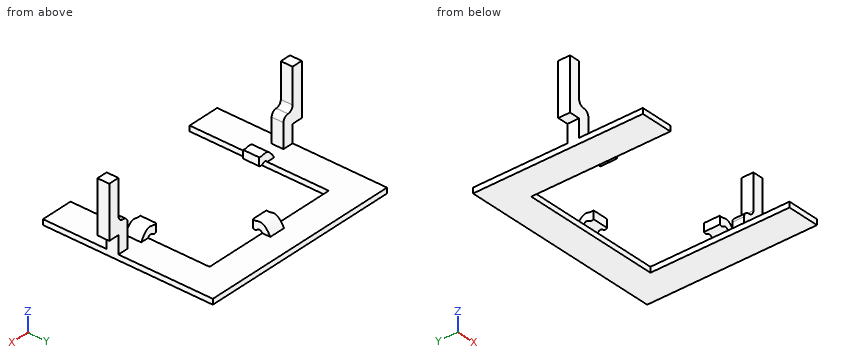
from build123d import *

# Parameters (mm, degrees)
BOSS_EXTRUDE1_DEPTH      = 1
BOSS_EXTRUDE2_START      = -1.5
BOSS_EXTRUDE2_DEPTH      = 3
CIRPATTERN1_COUNT        = 3
CIRPATTERN1_ANGLE        = 180
SKETCH4_W                = 2
SKETCH4_H                = 2.2
BOSS_EXTRUDE3_DEPTH      = 5.5
BOSS_EXTRUDE4_DEPTH      = 7.5
BOSS_EXTRUDE4_DEPTH_BACK = 2.2
SKETCH5_W                = 2
SKETCH5_H                = 2.2
FILLET1_START            = -30
FILLET1_DEPTH            = 4
FILLET1_START_2          = -29.415
FILLET1_2_DEPTH          = 2.2


with BuildPart() as part:
    # Sketch1 → Boss-Extrude1 (new body)
    with BuildSketch(Plane.XY):
        Polygon((13, -9.565), (-13, -9.565), (-19, -9.565), (-19, -41.315), (-13, -41.315), (-13, -15.315), (13, -15.315), (13, -41.315), (19, -41.315), (19, -9.565), align=None)
    extrude(amount=BOSS_EXTRUDE1_DEPTH)

    # Boss-Extrude2: read off the stored shape, not the designer's step
    # Boss-Extrude2 outline → Boss-Extrude2 (add)
    with BuildSketch(Plane(origin=(0, -28.315, 0), x_dir=(-1, 0, 0), z_dir=(0, -1, 0)).offset(BOSS_EXTRUDE2_START)):
        with BuildLine():
            Line((-11.23522271, -2.644286359), (-11.23522271, -1.144286359))
            add(Edge.make_bspline(
                [(-11.23522271, -1.144286359), (-11.740174878, -0.757764956), (-12.028679887, -1.161534837), (-12.227869222, -1.503002268), (-12.747184273, -1.488774458), (-13, -1)],
                knots=[0, 0, 0, 0, 0, 0, 1, 1, 1, 1, 1, 1], degree=5))
            Line((-13, -1), (-14.5, -1))
            add(Edge.make_bspline(
                [(-14.5, -1), (-13.760887065, -2.414906572), (-12.67824158, -3.40768712), (-12.345095428, -2.525951835), (-11.7215069, -2.450856602), (-11.23522271, -2.644286359)],
                knots=[0, 0, 0, 0, 0, 0, 1, 1, 1, 1, 1, 1], degree=5))
        make_face()
    boss_extrude2 = extrude(amount=BOSS_EXTRUDE2_DEPTH)

    # CirPattern1: Boss-Extrude2 ×3 about axis
    cirpattern1_axis = Axis((0, -28.315, 1.05), (0, 0, 1))
    for i in range(1, CIRPATTERN1_COUNT):
        add(boss_extrude2.rotate(cirpattern1_axis, i * CIRPATTERN1_ANGLE / (CIRPATTERN1_COUNT - 1)))

    # Sketch4 → Boss-Extrude3 (add)
    with BuildSketch(Plane.XY.offset(1)):
        with Locations((-18, -28.315)):
            Rectangle(SKETCH4_W, SKETCH4_H)
        with Locations((18, -28.315)):
            Rectangle(SKETCH4_W, SKETCH4_H)
    extrude(amount=BOSS_EXTRUDE3_DEPTH)

    # Sketch5 → Boss-Extrude4 (add, two sides: drawn at the far end of the back side and taken through both)
    with BuildSketch(Plane.XY.offset(6.5).offset(-BOSS_EXTRUDE4_DEPTH_BACK)):
        with Locations((-20, -28.315)):
            Rectangle(SKETCH5_W, SKETCH5_H)
        with Locations((20, -28.315)):
            Rectangle(SKETCH5_W, SKETCH5_H)
    extrude(amount=BOSS_EXTRUDE4_DEPTH + BOSS_EXTRUDE4_DEPTH_BACK)

    # Fillet1: read off the stored shape, not the designer's step
    # Fillet1 outline → Fillet1 (cut)
    with BuildSketch(Plane(origin=(0, 0, 0), x_dir=(1, 0, 0), z_dir=(0, 1, 0)).offset(FILLET1_START)):
        with BuildLine():
            Line((17, -6.5), (18, -6.5))
            ThreePointArc((18, -6.5), (17.292893219, -6.207106781), (17, -5.5))
            Line((17, -5.5), (17, -6.5))
        make_face()
        with BuildLine():
            ThreePointArc((-17, -5.5), (-17.292893219, -6.207106781), (-18, -6.5))
            Line((-18, -6.5), (-17, -6.5))
            Line((-17, -6.5), (-17, -5.5))
        make_face()
    extrude(amount=FILLET1_DEPTH, mode=Mode.SUBTRACT)

    # Fillet1 2 outline → Fillet1 2 (add)
    with BuildSketch(Plane(origin=(0, 0, 0), x_dir=(1, 0, 0), z_dir=(0, 1, 0)).offset(FILLET1_START_2)):
        with BuildLine():
            Line((19, -6.5), (18, -6.5))
            ThreePointArc((18, -6.5), (18.707106781, -6.792893219), (19, -7.5))
            Line((19, -7.5), (19, -6.5))
        make_face()
        with BuildLine():
            ThreePointArc((-19, -7.5), (-18.707106781, -6.792893219), (-18, -6.5))
            Line((-18, -6.5), (-19, -6.5))
            Line((-19, -6.5), (-19, -7.5))
        make_face()
    extrude(amount=FILLET1_2_DEPTH)


solid = part.part
Geometry: final body of the model. Coordinates: model frame, mm. Give positions to 0.01 mm unless a question says otherwise; leave off trailing zeros. Loops run counter-clockwise (first coordinate to the right, second up) from the corner with the lowest first, then second, coordinate; pieces in that order, holes last. Notation, with made-up numbers: M 77,79.25 L 101,79.25 A30 ccw 101,107.25 Z; hole C 47.5,-14 d2. An arc over 180 degrees is marked long. Put each result on its own line as item: value.
1) Material intervals for L1, parallel to X at y = -28.5, z = 5.5; L2, parallel to Z at x = 15, y = -18, sorted ascending. Write a range as from..to.
Computed values:
L1: x = -21..-17, 17..21
L2: z = 0..1
2) Cut plane B-B, the plane z = 8.75. Return the cut outline in (x, y) (3 decimals).
Computed values:
outline: M -21,-29.415 L -19,-29.415 L -19,-27.215 L -21,-27.215 Z; M 19,-29.415 L 21,-29.415 L 21,-27.215 L 19,-27.215 Z
3) Cut plane C-C, the plane x = -4. Return the cut outline in (y, z) (3 decimals), plus the area to 3 significant figures.
Computed values:
outline: M -15.315,0 L -9.565,0 L -9.565,1 L -15.315,1 Z
area: 5.75 mm^2
4) First-contact query: P1, Ø0.9, axis at x = -12, z = 1.5, coming from the +Y side (3 decimals); P2, Ø2, axis at x = -20, z = 5, coming from the +Y side (3 decimals); P3, Ø1.3, axis at y = -28, z = 2.5, coming from the +X side. Flat tips, straight axial feed; report the tip coordinate or a pass-through.
Computed values:
P1: stops at y = -26.815
P2: stops at y = -27.215
P3: stops at x = 19
5) Cut plane A-A, the plane y = -38. Return the cut outline in (x, z), plus the area to 3 significant figures.
Computed values:
outline: M -19,0 L -13,0 L -13,1 L -19,1 Z; M 13,0 L 19,0 L 19,1 L 13,1 Z
area: 12.0 mm^2
6) Cut plane D-D, the plane x = 15. Return the cut outline in (y, z) (3 decimals).
Computed values:
outline: M -41.315,0 L -9.565,0 L -9.565,1 L -41.315,1 Z
